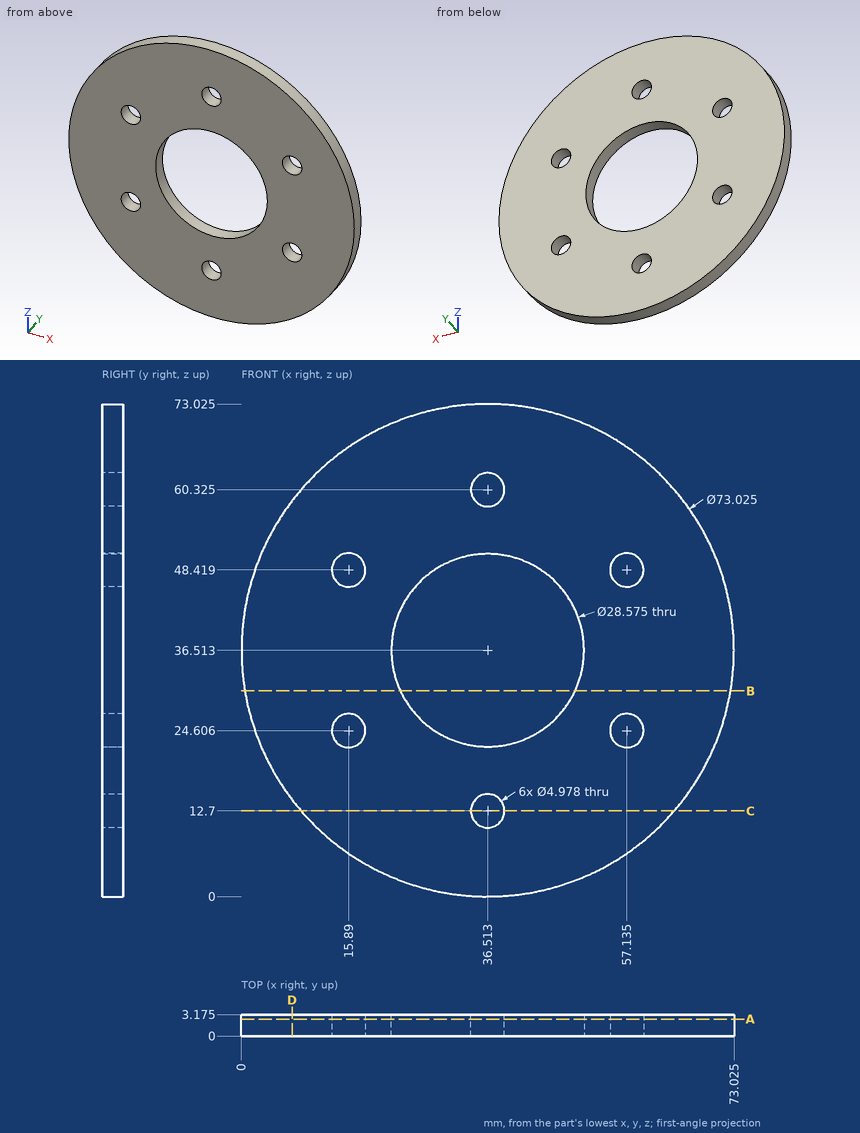
Answer from the drawing. Dimensions are ordinates in mm from the lowest x, y and z of the part. Round coordinates to 2 decimals unless told otherwise and drop trailing zeros. Write each loop counter-clockwise with the first axis right and the second up, starting at its lowest first coordinate (ties: lowest second). Pieces come first, ordered by that corner, then holes.
1. Given pin 1 Ø1 at (y, z) = (0.5, 31.5) entering from -X; pin 2 Ø1 at (x, y) = (15, 2.5) entering from +Z, each flat-ended and moving along its own axis, determine where each tip first touches the part or whether it passes through.
2. The part is cut by section D-D, the plane x = 7.5. Determine the outline of the cut face in (y, z) (1 decimal).
3. The part is cut by section B-B, the plane z = 30.5. Determine the outline of the cut face in (x, y) (1 decimal).
4. The part is cut by section A-A, the plane y = 2.5. State how many separate pieces and enclosed holes the cut face has, then the cut area to 3 significant figures.
5. The part is cut by section C-C, the plane z = 12.7. Determine the outline of the cut face in (x, y) (1 decimal).
6. Straight lines are drawn through the part: L1, parallel to Z at x = 36.5, y = 2.55 (1 decimal); L2, parallel to Z at x = 34.5, y = 1.2 (1 decimal); L3, parallel to Z at x = 16, y = 1.2 (1 decimal). For each, find the intervals that lie inside material, in ascending order.
Values:
1. pin 1: stops at x = 0.28
1. pin 2: stops at z = 66.37
2. outline: (0, 14.3) - (3.2, 14.3) - (3.2, 58.7) - (0, 58.7) - close
3. outline: (0.5, 0) - (23.6, 0) - (23.6, 3.2) - (0.5, 3.2) - close; (49.5, 0) - (72.5, 0) - (72.5, 3.2) - (49.5, 3.2) - close
4. separate pieces: 1
4. enclosed holes: 7
4. area: 3,430 mm2
5. outline: (8.8, 0) - (34, 0) - (34, 3.2) - (8.8, 3.2) - close; (39, 0) - (64.2, 0) - (64.2, 3.2) - (39, 3.2) - close
6. L1: z = 0 to 10.2, 15.2 to 22.2, 50.8 to 57.8, 62.8 to 73
6. L2: z = 0.1 to 11.2, 14.2 to 22.4, 50.7 to 58.9, 61.8 to 73
6. L3: z = 6.3 to 22.1, 27.1 to 45.9, 50.9 to 66.7
